CAD build for the part. Positions are in the model's coordinates, mm. Face numbers are marked on the shaded views. Give positions to 0.01 mm unless a question says otherwise; leave off trailing zeros. Loops run counter-clockwise (first coordinate to the right, second up) from the corner with the lowest first, then second, coordinate; pieces in that order, holes last.
Item 1: Saw through at A-A on z = 3. Give the cut face in (x, y) (3 decimals).
Item 2: Drop flat-ended pins along their axis: P1, Ø1, axis at x = 25, z = 2.5, coming from the +Y side; P2, Ø1, axis at y = -9.5, z = 5.5, coming from the +X side; P3, Ø1.5, axis at x = 8, z = 2, coming from the -Y side. Give the stop position or say it passes through.
Item 3: Saw through at C-C on x = 10. Give the cut face in (y, z).
Item 4: Mould opens along Y. For the marked faces 1, 2 and 3 say: released by +Y, released by -Y, zero draft, split by the parting line, or undercut.
Item 5: Saw through at D-D on y = -4.75. Give the cut face in (x, z), plus the area to 3 significant figures.
Item 6: Probe probe 1 along Y at (x, z) = (-30, 3) (3 decimals); probe 2 along Y at (x, z) = (0, 2.5) (3 decimals); probe 3 along X at (y, z) = (-8.5, 0.5). List the from-to ranges inside material, lowest first.
Item 7: Saw through at B-B on y = 0. Give the cut face in (x, z) (3 decimals), plus the area to 3 significant figures.
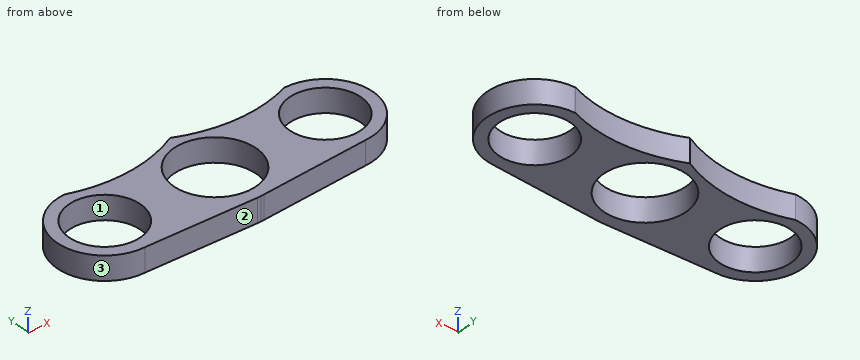
from build123d import *

# Parameters (mm, degrees)
F0_R     = 9.55
F1_DEPTH = 6.35
F3_DEPTH = 25


# Not quite as in the source:
# - a feature names something its author has since deleted; it is built from what else it names


with BuildPart() as f1:
    # F0 (on Top) → F1 (new body)
    with BuildSketch(Plane.XY):
        with BuildLine():
            Line((14.175, 0), (11, 0))
            ThreePointArc((11, 0), (0, -11), (-11, 0))
            Line((-11, 0), (-14.175, 0))
            ThreePointArc((-14.175, 0), (-10.265086005, -9.7754096748), (-0.6923002736, -14.1580840982))
            ThreePointArc((-0.6923002736, -14.1580840982), (-0.2241695179, -14.1732273328), (0.2442059858, -14.1728962614))
            Line((0.2442059858, -14.1728962614), (1.1329762166, -14.1296493195))
            ThreePointArc((1.1329762166, -14.1296493195), (10.4161068272, -9.6143301152), (14.175, 0))
        make_face()
        with BuildLine():
            ThreePointArc((-11, 0), (0, 11), (11, 0))
            Line((11, 0), (14.175, 0))
            ThreePointArc((14.175, 0), (10.4954430476, 9.5276597459), (1.3670564043, 14.1089256071))
            Line((1.3670564043, 14.1089256071), (0, 14.175))
            Line((0, 14.175), (-1.3670564043, 14.1089256071))
            ThreePointArc((-1.3670564043, 14.1089256071), (-10.4954430476, 9.5276597459), (-14.175, 0))
            Line((-14.175, 0), (-11, 0))
        make_face()
        with BuildLine():
            Line((17.275, 0), (14.175, 0))
            ThreePointArc((14.175, 0), (10.4161068272, -9.6143301152), (1.1329762166, -14.1296493195))
            Line((1.1329762166, -14.1296493195), (30, -12.725))
            ThreePointArc((30, -12.725), (21.0020662094, -8.9979337906), (17.275, 0))
        make_face()
        with BuildLine():
            ThreePointArc((1.3670564043, 14.1089256071), (10.4954430476, 9.5276597459), (14.175, 0))
            Line((14.175, 0), (17.275, 0))
            ThreePointArc((17.275, 0), (21.0020662094, 8.9979337906), (30, 12.725))
            Line((30, 12.725), (1.3670564043, 14.1089256071))
        make_face()
        with BuildLine():
            Line((-17.275, 0), (-14.175, 0))
            ThreePointArc((-14.175, 0), (-10.4954430476, 9.5276597459), (-1.3670564043, 14.1089256071))
            Line((-1.3670564043, 14.1089256071), (-30, 12.725))
            ThreePointArc((-30, 12.725), (-21.0020662094, 8.9979337906), (-17.275, 0))
        make_face()
        with BuildLine():
            ThreePointArc((-0.6923002736, -14.1580840982), (-10.265086005, -9.7754096748), (-14.175, 0))
            Line((-14.175, 0), (-17.275, 0))
            ThreePointArc((-17.275, 0), (-21.0020662094, -8.9979337906), (-30, -12.725))
            Line((-30, -12.725), (-0.6923002736, -14.1580840982))
        make_face()
        with BuildLine():
            ThreePointArc((30, 12.725), (21.0020662094, 8.9979337906), (17.275, 0))
            ThreePointArc((17.275, 0), (21.0020662094, -8.9979337906), (30, -12.725))
            ThreePointArc((30, -12.725), (38.9979337906, -8.9979337906), (42.725, 0))
            ThreePointArc((42.725, 0), (38.9979337906, 8.9979337906), (30, 12.725))
        make_face()
        with BuildLine():
            ThreePointArc((39.55, 0), (30, -9.55), (20.45, 0))
            ThreePointArc((20.45, 0), (30, 9.55), (39.55, 0))
        make_face(mode=Mode.SUBTRACT)
        with BuildLine():
            ThreePointArc((-30, -12.725), (-21.0020662094, -8.9979337906), (-17.275, 0))
            ThreePointArc((-17.275, 0), (-21.0020662094, 8.9979337906), (-30, 12.725))
            ThreePointArc((-30, 12.725), (-42.725, 0), (-30, -12.725))
        make_face()
        with Locations((-30, 0)):
            Circle(F0_R, mode=Mode.SUBTRACT)
    extrude(amount=F1_DEPTH)

    # F2 (on Top) → F3 (cut)
    with BuildSketch(Plane.XY):
        with BuildLine():
            ThreePointArc((-0.0002806461, 14.1748610267), (-20.9243917712, 47.820811609), (-0.0002806461, 81.4667621913))
            ThreePointArc((-0.0002806461, 81.4667621913), (-54.2064032082, 47.820811609), (-0.0002806461, 14.1748610267))
        make_face()
        with BuildLine():
            ThreePointArc((-0.0002806461, 14.1748610267), (15.2384059917, 28.0205677125), (20.8838914193, 47.820811609))
            ThreePointArc((20.8838914193, 47.820811609), (15.2384059917, 67.6210555055), (-0.0002806461, 81.4667621913))
            ThreePointArc((-0.0002806461, 81.4667621913), (-20.9243917712, 47.820811609), (-0.0002806461, 14.1748610267))
        make_face()
        with BuildLine():
            ThreePointArc((-0.0002806461, 81.4667621913), (15.2384059917, 67.6210555055), (20.8838914193, 47.820811609))
            ThreePointArc((20.8838914193, 47.820811609), (15.2384059917, 28.0205677125), (-0.0002806461, 14.1748610267))
            ThreePointArc((-0.0002806461, 14.1748610267), (36.3997744183, 15.9650923463), (54.1023755584, 47.820811609))
            ThreePointArc((54.1023755584, 47.820811609), (36.3997744183, 79.6765308717), (-0.0002806461, 81.4667621913))
        make_face()
    extrude(amount=F3_DEPTH, mode=Mode.SUBTRACT)


solid = f1.part
Results below:
1. outline: (-30, -12.725) - (-0.692, -14.158) arc R14.175 ccw to (0.244, -14.173) - (30, -12.725) arc R12.725 ccw to (30, 12.725) - (29.856, 12.732) arc R37.513 cw to (0, 14.175) arc R37.545 cw to (-30, 12.725) arc R12.725 ccw to start; hole circle Ø19.1 at (-30, 0); hole circle Ø22 at (0, 0); hole circle Ø19.1 at (30, 0)
2. P1: stops at y = 11.38
2. P2: stops at x = 39
2. P3: stops at y = -13.83
3. outline: (-13.7, 0) - (-4.58, 0) - (-4.58, 6.35) - (-13.7, 6.35) - close; (4.58, 0) - (10.89, 0) - (10.89, 6.35) - (4.58, 6.35) - close
4. face 1: undercut
4. face 2: released by -Y
4. face 3: split by the parting line
5. outline: (-41.81, 0) - (-38.28, 0) - (-38.28, 6.35) - (-41.81, 6.35) - close; (-21.72, 0) - (-9.92, 0) - (-9.92, 6.35) - (-21.72, 6.35) - close; (9.92, 0) - (21.72, 0) - (21.72, 6.35) - (9.92, 6.35) - close; (38.28, 0) - (41.81, 0) - (41.81, 6.35) - (38.28, 6.35) - close
5. area: 194 mm2
6. probe 1: y = -12.725 to -9.55, 9.55 to 12.725
6. probe 2: y = -14.175 to -11, 11 to 14.175
6. probe 3: x = -39.47 to -34.35, -25.65 to -6.98, 6.98 to 25.65, 34.35 to 39.47
7. outline: (-42.725, 0) - (-39.55, 0) - (-39.55, 6.35) - (-42.725, 6.35) - close; (-20.45, 0) - (-11, 0) - (-11, 6.35) - (-20.45, 6.35) - close; (11, 0) - (20.45, 0) - (20.45, 6.35) - (11, 6.35) - close; (39.55, 0) - (42.725, 0) - (42.725, 6.35) - (39.55, 6.35) - close
7. area: 160 mm2
